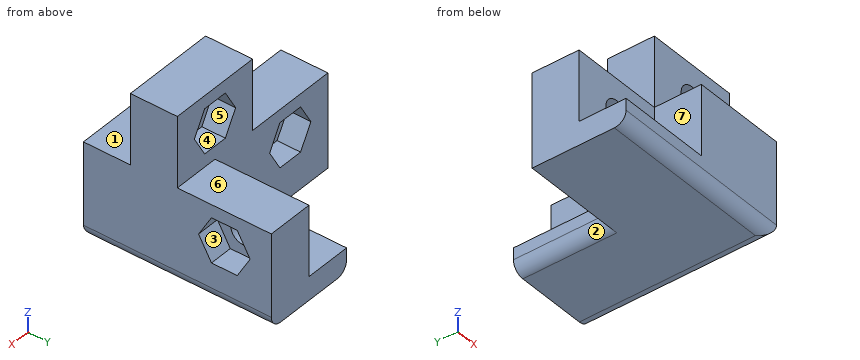
Autodesk Inventor part; units mm, degrees
ref_plane "YZ Plane" through (0, 0, 0) normal (1, 0, 0) x (0, 1, 0)
ref_plane "XZ Plane" through (0, 0, 0) normal (0, 1, 0) x (-1, 0, 0)
ref_plane "XY Plane" through (0, 0, 0) normal (0, 0, 1) x (1, 0, 0)
sketch "Sketch1" plane through (0, 0, 0) normal (0, 0, 1) x (1, 0, 0)
  line L0 (0, 0) -> (12, 0)
  line L1 (12, 0) -> (12, 12)
  line L2 (12, 12) -> (0, 12)
  line L3 (0, 12) -> (0, 0)
  line L4 (12, 0) -> (0, 0)
  line L5 (0, 0) -> (0, -12)
  line L6 (0, -12) -> (12, -12)
  line L7 (12, -12) -> (12, 0)
  line L8 (12, 0) -> (24, 0)
  line L9 (24, 0) -> (24, -12)
  line L10 (24, -12) -> (12, -12)
  line L11 (12, -12) -> (12, 0)
  line L12 (0, -12) -> (-12, -12)
  line L13 (-12, -12) -> (-12, 0)
  line L14 (-12, 0) -> (0, 0)
  line L15 (0, 0) -> (0, -12)
  line L16 (0, -12) -> (12, -12)
  line L17 (12, -12) -> (12, -24)
  line L18 (12, -24) -> (0, -24)
  line L19 (0, -24) -> (0, -12)
  dimension "d0" = 12
  dimension "d1" = 12
  dimension "d2" = 12
  dimension "d3" = 12
  dimension "d4" = 12
  dimension "d5" = 12
  dimension "d6" = 12
  dimension "d7" = 12
  dimension "d8" = 12
  dimension "d9" = 12
extrude "Extrusion1" add sketch "Sketch1" along normal blind 3
sketch "Sketch2" plane through (0, 0, 3) normal (0, 0, 1) x (1, 0, 0)
  line L0 (-12, 0) -> (-12, -12)
  line L1 (-12, -12) -> (-12, -6)
  line L2 (-12, -6) -> (0, -6)
  line L3 (-12, -12) -> (0, -12)
  line L4 (0, -6) -> (0, -12)
  line L5 (0, -12) -> (-12, -12)
  line L6 (12, -24) -> (12, -12)
  line L7 (12, -12) -> (12, -6)
  line L8 (12, -6) -> (24, -6)
  line L9 (24, -12) -> (24, 0)
  line L10 (12, -12) -> (24, -12)
  line L11 (24, -6) -> (24, -12)
  line L12 (24, -12) -> (12, -12)
  line L13 (0, 0) -> (0, -6)
  line L14 (12, 0) -> (12, 12)
  line L15 (0, 0) -> (12, 0)
  line L16 (12, 0) -> (12, -6)
  line L17 (12, -12) -> (0, -12)
  line L18 (0, 12) -> (0, 0)
  line L19 (0, 0) -> (0, 12)
  line L20 (0, 12) -> (6, 12)
  line L21 (12, 12) -> (0, 12)
  line L22 (6, 12) -> (6, 0)
  line L23 (6, 0) -> (0, 0)
  line L24 (0, -12) -> (0, -24)
  line L25 (0, -12) -> (0, -24)
  line L26 (0, -24) -> (6, -24)
  line L27 (0, -24) -> (12, -24)
  line L28 (6, -24) -> (6, -12)
  line L29 (6, -12) -> (0, -12)
  dimension "d12" = 6
  dimension "d13" = 12
extrude "Extrusion2" add sketch "Sketch2" along normal blind 9 contours L2 L4 L3 L0 | L13 L15 L16 L7 L17 L4 | L17 L28 L26 L24 | L18 L20 L22 L15 | L7 L8 L9 L10
sketch "Sketch3" plane through (0, 0, 12) normal (0, 0, 1) x (1, 0, 0)
  line L0 (0, -6) -> (12, -6)
  line L1 (12, -12) -> (6, -12)
  line L2 (12, -6) -> (12, -12)
  line L3 (0, -12) -> (0, -24)
  line L4 (12, -12) -> (0, -12)
  line L5 (0, -12) -> (0, -6)
  point P0 (0, 0)
extrude "Extrusion3" add sketch "Sketch3" along normal blind 9
sketch "Sketch4" plane through (6, -12, 3) normal (0, -1, 0) x (1, 0, 0)
  point P0 (-6, -3)
sketch "Sketch5" plane through (-12, -6, 3) normal (0, 1, 0) x (1, 0, 0)
  circle A0 centre (6, -4.5) radius 1.725
  line L0 (0, 0) -> (0, -9)
  line L1 (12, -9) -> (0, -9)
  circle A1 centre (18, -13.5) radius 1.725
  line L2 (24, -18) -> (12, -18)
  line L3 (24, -9) -> (24, -18)
  circle A2 centre (30, -4.5) radius 1.725
  line L4 (36, 0) -> (36, -9)
  line L5 (36, -9) -> (24, -9)
  point P0 (12, 3)
  dimension "d19" = 3.45
  dimension "d20" = 6
  dimension "d21" = 4.5
  dimension "d22" = 3.45
  dimension "d23" = 4.5
  dimension "d24" = 6
  dimension "d25" = 3.45
  dimension "d26" = 6
  dimension "d27" = 4.5
extrude "Extrusion4" cut sketch "Sketch5" against normal blind 3
sketch "Sketch6" plane through (6, -12, 3) normal (0, -1, 0) x (1, 0, 0)
  circle A0 centre (-12, 4.5) radius 1.725
  line L0 (-10.3546, 7.35) -> (-8.7091, 4.5)
  line L1 (-8.7091, 4.5) -> (-10.3546, 1.65)
  line L2 (-10.3546, 1.65) -> (-13.6454, 1.65)
  line L3 (-13.6454, 1.65) -> (-15.2909, 4.5)
  line L4 (-15.2909, 4.5) -> (-13.6454, 7.35)
  line L5 (-13.6454, 7.35) -> (-10.3546, 7.35)
  circle A1 centre (12, 4.5) radius 1.725
  line L6 (13.6454, 7.35) -> (15.2909, 4.5)
  line L7 (15.2909, 4.5) -> (13.6454, 1.65)
  line L8 (13.6454, 1.65) -> (10.3546, 1.65)
  line L9 (10.3546, 1.65) -> (8.7091, 4.5)
  line L10 (8.7091, 4.5) -> (10.3546, 7.35)
  line L11 (10.3546, 7.35) -> (13.6454, 7.35)
  circle A2 centre (0, 13.5) radius 1.725
  line L12 (1.6454, 16.35) -> (3.2909, 13.5)
  line L13 (3.2909, 13.5) -> (1.6454, 10.65)
  line L14 (1.6454, 10.65) -> (-1.6454, 10.65)
  line L15 (-1.6454, 10.65) -> (-3.2909, 13.5)
  line L16 (-3.2909, 13.5) -> (-1.6454, 16.35)
  line L17 (-1.6454, 16.35) -> (1.6454, 16.35)
  point P0 (-6, -3)
  dimension "d30" = 2.85
  dimension "d31" = 2.85
  dimension "d32" = 2.85
extrude "Extrusion5" cut sketch "Sketch6" against normal blind 3 contours A0 | L0 L1 L2 L3 L4 L5 | A1 | L6 L7 L8 L9 L10 L11 | A2 | L12 L13 L14 L15 L16 L17
sketch "Sketch7" plane through (6, 0, 3) normal (1, 0, 0) x (0, 0, -1)
  circle A0 centre (-4.5, 6) radius 1.725
  circle A1 centre (-4.5, -18) radius 1.725
  line L0 (-9, 0) -> (-9, 12)
  line L1 (-9, -24) -> (-9, -12)
  line L2 (0, -24) -> (-9, -24)
  line L3 (0, 12) -> (-9, 12)
  point P0 (3, 0)
  dimension "d35" = 3.45
  dimension "d36" = 3.45
  dimension "d37" = 4.5
  dimension "d38" = 4.5
  dimension "d39" = 6
  dimension "d40" = 6
extrude "Extrusion6" cut sketch "Sketch7" against normal blind 3
sketch "Sketch8" plane through (0, -6, 3) normal (-1, 0, 0) x (0, 0, 1)
  circle A0 centre (4.5, 12) radius 1.725
  line L0 (1.65, 13.6454) -> (4.5, 15.2909)
  line L1 (4.5, 15.2909) -> (7.35, 13.6454)
  line L2 (7.35, 13.6454) -> (7.35, 10.3546)
  line L3 (7.35, 10.3546) -> (4.5, 8.7091)
  line L4 (4.5, 8.7091) -> (1.65, 10.3546)
  line L5 (1.65, 10.3546) -> (1.65, 13.6454)
  circle A1 centre (4.5, -12) radius 1.725
  line L6 (1.65, -10.3546) -> (4.5, -8.7091)
  line L7 (4.5, -8.7091) -> (7.35, -10.3546)
  line L8 (7.35, -10.3546) -> (7.35, -13.6454)
  line L9 (7.35, -13.6454) -> (4.5, -15.2909)
  line L10 (4.5, -15.2909) -> (1.65, -13.6454)
  line L11 (1.65, -13.6454) -> (1.65, -10.3546)
  point P0 (-3, 6)
  dimension "d43" = 2.85
  dimension "d44" = 2.85
extrude "Extrusion7" cut sketch "Sketch8" against normal blind 3 contours A0 | L0 L1 L2 L3 L4 L5 | A1 | L6 L7 L8 L9 L10 L11
sketch "Sketch9" plane through (0, 0, 0) normal (0, 0, -1) x (-1, 0, 0)
  line L0 (-24, -12) -> (-24, 0)
  line L1 (-12, -12) -> (-12, -6)
  line L2 (-24, 0) -> (-12, 0)
  line L3 (-12, 0) -> (-12, -12)
  line L4 (-12, -12) -> (-24, -12)
  line L5 (-24, -12) -> (-24, 0)
  line L6 (-12, -12) -> (0, -12)
  line L7 (0, -12) -> (0, -24)
  line L8 (0, -24) -> (-12, -24)
  line L9 (-12, -24) -> (-12, -12)
  point P0 (0, 0)
extrude "Extrusion8" cut sketch "Sketch9" against normal through all
sketch "Sketch10" plane through (0, 12, 12) normal (0, 1, 0) x (1, 0, 0)
  line L0 (6, 0) -> (0, 0)
  line L1 (12, 9) -> (6, 9)
  line L2 (0, 0) -> (6, 0)
  line L3 (6, 0) -> (6, 9)
  line L4 (6, 9) -> (0, 9)
  line L5 (0, 9) -> (0, 0)
  point P0 (0, 12)
extrude "Extrusion9" cut sketch "Sketch10" against normal blind 12
sketch "Sketch11" plane through (0, 0, 3) normal (0, 1, 0) x (1, 0, 0)
  line L0 (12, 0) -> (12, -9)
  line L1 (12, 0) -> (0, 0)
  line L2 (12, -9) -> (6, -9)
  line L3 (6, -9) -> (6, 0)
  line L4 (6, 0) -> (12, 0)
  line L5 (12, 0) -> (12, -9)
  point P0 (0, 3)
extrude "Extrusion10" add sketch "Sketch11" along normal blind 12
sketch "Sketch12" plane through (6, 0, 3) normal (-1, 0, 0) x (0, 0, 1)
  circle A0 centre (4.5, 6) radius 1.575
  line L0 (9, 0) -> (9, 12)
  line L1 (0, 12) -> (9, 12)
  point P0 (-3, 0)
  dimension "d54" = 3.15
  dimension "d55" = 4.5
  dimension "d56" = 6
extrude "Extrusion11" cut sketch "Sketch12" against normal blind 3
sketch "Sketch13" plane through (12, -6, 12) normal (1, 0, 0) x (0, 0, -1)
  circle A0 centre (4.5, 12) radius 1.575
  line L0 (1.65, 13.6454) -> (4.5, 15.2909)
  line L1 (4.5, 15.2909) -> (7.35, 13.6454)
  line L2 (7.35, 13.6454) -> (7.35, 10.3546)
  line L3 (7.35, 10.3546) -> (4.5, 8.7091)
  line L4 (4.5, 8.7091) -> (1.65, 10.3546)
  line L5 (1.65, 10.3546) -> (1.65, 13.6454)
  point P0 (12, 6)
  dimension "d59" = 5.7
extrude "Extrusion12" cut sketch "Sketch13" against normal blind 3 contours A0 | L0 L1 L2 L3 L4 L5
sketch "Sketch14" plane through (0, -6, 3) normal (-1, 0, 0) x (0, 0, 1)
  line L0 (9, 6) -> (0, 6)
  line L1 (0, 6) -> (0, 0)
  line L2 (9, 6) -> (0, 6)
  line L3 (0, 6) -> (0, 0)
  line L4 (0, 0) -> (9, 0)
  line L5 (9, 0) -> (9, 6)
  point P0 (-3, 6)
extrude "Extrusion13" add sketch "Sketch14" along normal blind 12
sketch "Sketch15" plane through (-12, -12, 0) normal (-1, 0, 0) x (0, 0, 1)
  line L0 (12, 0) -> (12, 6)
  line L1 (12, 0) -> (3, 0)
  line L2 (3, 0) -> (3, 6)
  line L3 (3, 6) -> (12, 6)
  line L4 (12, 6) -> (12, 0)
  point P0 (0, 12)
  dimension "d64" = 9
  dimension "d65" = 6
extrude "Extrusion14" cut sketch "Sketch15" against normal blind 12
sketch "Sketch16" plane through (-12, -6, 12) normal (0, -1, 0) x (1, 0, 0)
  circle A0 centre (6, -4.5) radius 1.725
  line L0 (0, -9) -> (0, 0)
  line L1 (0, 0) -> (12, 0)
  point P0 (12, -12)
  dimension "d68" = 3.45
  dimension "d69" = 6
  dimension "d70" = 4.5
extrude "Extrusion15" cut sketch "Sketch16" against normal blind 3
sketch "Sketch17" plane through (-12, 0, 0) normal (0, 1, 0) x (1, 0, 0)
  circle A0 centre (6, -7.5) radius 1.725
  line L0 (4.3546, -10.35) -> (2.7091, -7.5)
  line L1 (2.7091, -7.5) -> (4.3546, -4.65)
  line L2 (4.3546, -4.65) -> (7.6454, -4.65)
  line L3 (7.6454, -4.65) -> (9.2909, -7.5)
  line L4 (9.2909, -7.5) -> (7.6454, -10.35)
  line L5 (7.6454, -10.35) -> (4.3546, -10.35)
  point P0 (12, 0)
  dimension "d73" = 5.7
extrude "Extrusion16" cut sketch "Sketch17" against normal blind 3 contours A0 | L0 L1 L2 L3 L4 L5
sketch "Sketch18" plane through (0, 0, 12) normal (0, 0, 1) x (1, 0, 0)
  line L0 (12, -6) -> (12, 12)
  line L1 (0, 0) -> (12, 0)
  line L2 (12, 0) -> (12, -6)
  line L3 (12, -6) -> (0, -6)
  line L4 (0, -6) -> (0, 0)
extrude "Extrusion17" add sketch "Sketch18" along normal blind 9
sketch "Sketch19" plane through (0, 0, 21) normal (0, 0, 1) x (1, 0, 0)
  line L0 (0, -12) -> (12, -12)
  line L1 (12, -12) -> (12, 0)
  line L2 (0, -12) -> (12, -12)
  line L3 (12, -12) -> (12, -6)
  line L4 (12, -6) -> (0, -6)
  line L5 (0, -6) -> (0, -12)
  point P0 (0, 0)
extrude "Extrusion18" cut sketch "Sketch19" against normal blind 9
sketch "Sketch20" plane through (0, -6, 21) normal (0, -1, 0) x (1, 0, 0)
  circle A0 centre (6, -4.5) radius 1.725
  line L0 (0, 0) -> (12, 0)
  line L1 (0, -9) -> (0, 0)
  point P0 (0, -21)
  dimension "d80" = 3.45
  dimension "d81" = 4.5
  dimension "d82" = 6
extrude "Extrusion19" cut sketch "Sketch20" against normal blind 3
sketch "Sketch21" plane through (-12, 0, 0) normal (0, 1, 0) x (1, 0, 0)
  circle A0 centre (18, -16.5) radius 1.725
  line L0 (16.3546, -19.35) -> (14.7091, -16.5)
  line L1 (14.7091, -16.5) -> (16.3546, -13.65)
  line L2 (16.3546, -13.65) -> (19.6454, -13.65)
  line L3 (19.6454, -13.65) -> (21.2909, -16.5)
  line L4 (21.2909, -16.5) -> (19.6454, -19.35)
  line L5 (19.6454, -19.35) -> (16.3546, -19.35)
  point P0 (12, 0)
  dimension "d85" = 5.7
extrude "Extrusion20" cut sketch "Sketch21" against normal blind 3 contours A0 | L0 L1 L2 L3 L4 L5
fillet "Fillet3" radius 1.5 3 edges at (0, -12, 0) (12, 0, 0) (0, 6, 0)
properties part number "topCornSW"
Source: CAD feature listing. Evaluate the final solid. Frame: model axes, mm. Face numbers are marked on the shaded views. A direction names the side the tool comes from. Give positions to 0.01 mm unless a question says otherwise; leave off trailing zeros. Loops run counter-clockwise (first coordinate to the right, second up) from the corner with the lowest first, then second, coordinate; pieces in that order, holes last. Notation, with made-up numbers: (4.25, 71.5) - (32.25, 71.5) arc R22 ccw to (32.25, 104.5) - close; hole circle Ø8 at (-3, -9.75). An arc over 180 degrees is marked (long way). Use CSV: the item, a comma, the result in double quotes. Start each with the question number.
1. Reachability of the marked faces 1, 2, 3 and 4 from +Z, -Z, +X, -X, +Y, -Y: full face, straight path, thin tool, end or side. Return the list, or none.
2. Ray query, L1, parallel to Y at x = 8.2, z = 7.5 (3 decimals); L2, parallel to Y at x = -7.25, z = 9; L3, parallel to X at y = -2.25, z = 16. Return the intervals inside material, ascending.
3. Section A-A (x = -6). Output: boundary loops of the cut face in (y, z) (3 decimals), then the cut area to 3 significant figures.
4. Draft query along Z for the marked faces 5, 6 and 7. Return one class per face: +Z half, -Z half, draft (parallel to the pull), parting line (faces both ways), or undercut.
5. Pin query (flat end, axial travel): pin 1 (1.6 mm diameter, centred on y = 5.5, z = 2, fed in from -X); pin 2 (5 mm diameter, centred on x = 8.5, y = 7, fed in from +Z); pin 3 (5.5 mm diameter, centred on x = -6, z = 7.5, fed in from +Y). Return the tip coordinate at first contact, or that it passes through.
6. Section B-B (y = 6). Output: boundary loops of the cut face in (x, z) (3 decimals), then the cut area to 3 significant figures.
7. Section D-D (y = 0.5). Output: boundary loops of the cut face in (x, z), then the cut area to 3 significant figures.
8. Section C-C (z = 16). Output: boundary loops of the cut face in (x, y), then the cut area to 3 significant figures.
Response:
1,face 1,"+Z, +X, -X, -Y"
1,face 2,"-Z, -X, +Y"
1,face 3,"+X"
1,face 4,"+Y"
2,L1,"-12 to 4.425, 7.575 to 12"
2,L2,"-6 to -3"
2,L3,"0 to 3, 9 to 12"
3,outline,"(-12, 1.5) arc R1.5 ccw to (-10.5, 0) - (0, 0) - (0, 4.65) - (-3, 4.65) - (-3, 5.775) - (-6, 5.775) - (-6, 3) - (-12, 3) - close; (-6, 9.225) - (-3, 9.225) - (-3, 10.35) - (0, 10.35) - (0, 12) - (-6, 12) - close"
3,area,"62.1 mm²"
4,face 5,"undercut"
4,face 6,"+Z half"
4,face 7,"draft"
5,pin 1,"x = 0"
5,pin 2,"z = 12"
5,pin 3,"y = -3"
6,outline,"(0, 1.5) arc R1.5 ccw to (1.5, 0) - (10.5, 0) arc R1.5 ccw to (12, 1.5) - (12, 4.65) - (9, 4.65) - (9, 5.925) - (6, 5.925) - (6, 3) - (0, 3) - close; (6, 9.075) - (9, 9.075) - (9, 10.35) - (12, 10.35) - (12, 12) - (6, 12) - close"
6,area,"62.5 mm²"
7,outline,"(0, 1.5) arc R1.5 ccw to (1.5, 0) - (10.5, 0) arc R1.5 ccw to (12, 1.5) - (12, 12) - (6, 12) - (6, 3) - (0, 3) - close"
7,area,"89.0 mm²"
8,outline,"(0, -6) - (4.35, -6) - (4.35, -3) - (3, -3) - (3, 0) - (0, 0) - close; (7.65, -6) - (12, -6) - (12, 0) - (9, 0) - (9, -3) - (7.65, -3) - close"
8,area,"44.1 mm²"
